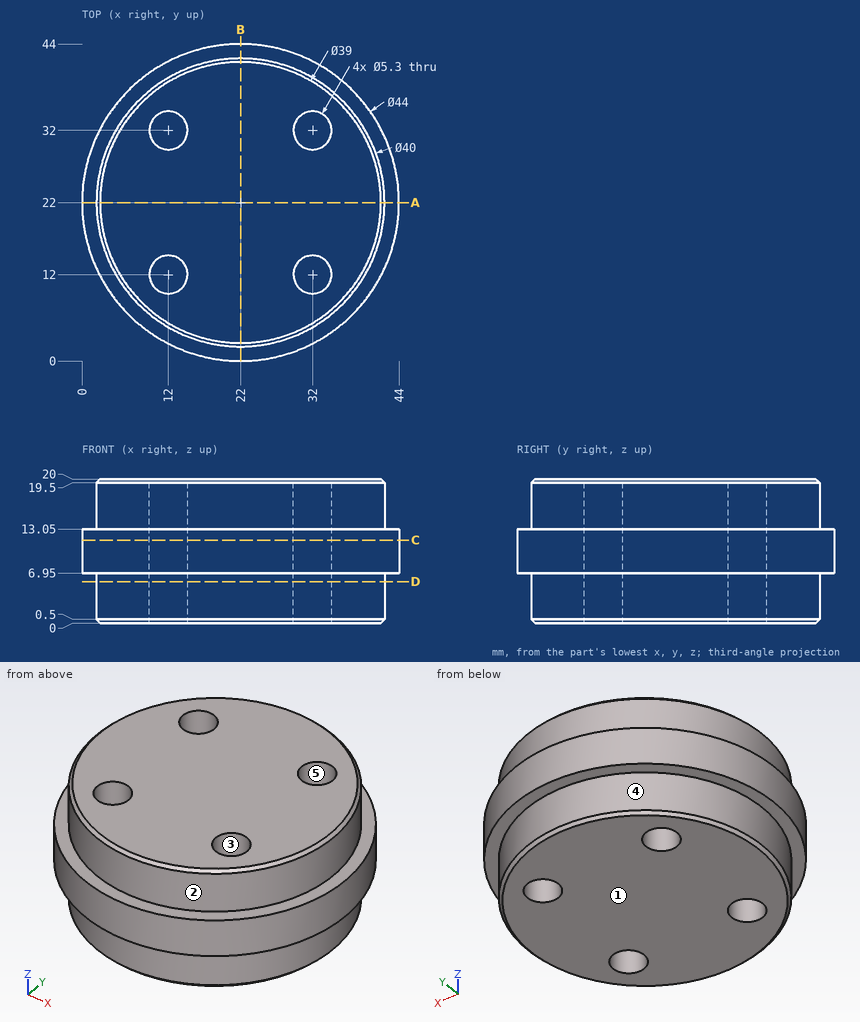
For this review, use the dimensioned drawing (mm, ordinates from the lowest corner) and the shaded views. A direction names the side the tool comes from. Round coordinates to 2 decimals unless told otherwise and drop trailing zeros. Order: outer loops, then holes, each group sorted by start corner. A loop starts at its lowest first (then second) coordinate and runs counter-clockwise, first axis right, second up. Notation, with made-up numbers: M 33,-11.75 L 78,-11.75 A7 ccw 78,-1.75 Z; hole C -22,54.5 d2. An arc over 180 degrees is marked long. Use a Markdown table: item, result.
1) Wall thickness on line 1 along X through (y, z) = (11.5, 11); line 2 along X through (y, z) = (12, 6); line 3 along Y through (x, z) = (12, 9.5): over which ranges is each line inside the solid? List them lowest first. Write a range as [from, to].
Report:
| item | result |
|---|---|
| line 1 | [2.67, 9.4], [14.6, 29.4], [34.6, 41.33] |
| line 2 | [4.68, 9.35], [14.65, 29.35], [34.65, 39.32] |
| line 3 | [2.4, 9.35], [14.65, 29.35], [34.65, 41.6] |
2) Consider section C-C (z = 11.5). Write out the cut boundary in (x, y).
Report:
| item | result |
|---|---|
| outline | C 22,22 d44; hole C 12,12 d5.3; hole C 12,32 d5.3; hole C 32,12 d5.3; hole C 32,32 d5.3 |
3) Draft analysis for pull direction Y (two halves, no side actions). For the marked faces 1, 2 and 3, state which applies: released by +Y, released by -Y, zero draft, split by the parting line, or undercut.
Report:
| item | result |
|---|---|
| face 1 | zero draft |
| face 2 | split by the parting line |
| face 3 | undercut |
4) Consider section A-A (y = 22). Write out the cut boundary in (x, z).
Report:
| item | result |
|---|---|
| outline | M 0,6.95 L 2,6.95 L 2,0.5 L 2.5,0 L 41.5,0 L 42,0.5 L 42,6.95 L 44,6.95 L 44,13.05 L 42,13.05 L 42,19.5 L 41.5,20 L 2.5,20 L 2,19.5 L 2,13.05 L 0,13.05 Z |
5) Tool access review of the marked faces 4 and 5: name each direction out of +Z, -Z, +X, -X, +Y, -Y from which nothing blocks a thin tool from reaching the whole face with its end or side.
Report:
| item | result |
|---|---|
| face 4 | -Z |
| face 5 | +Z, -Z |
6) Consider section D-D (z = 5.75). Write out the cut boundary in (x, y).
Report:
| item | result |
|---|---|
| outline | C 22,22 d40; hole C 12,12 d5.3; hole C 12,32 d5.3; hole C 32,12 d5.3; hole C 32,32 d5.3 |
7) Insertion check: pin 1 (1 mm diameter, centred on x = 12, z = 10, fed in from +Y); pin 2 (2 mm diameter, centred on y = 26.5, z = 14.5, fed in from +X); pin 3 (5 mm diameter, centred on y = 12, z = 3, fed in from -X). Each pin has a flat end and moves straight along its axis. Give the tip position at first contact, or say it passes through.
Report:
| item | result |
|---|---|
| pin 1 | y = 41.84 |
| pin 2 | x = 41.69 |
| pin 3 | x = 3.46 |
